Source: CAD feature listing. Evaluate the final solid. Frame: model axes, mm. A direction names the side the tool comes from. Give positions to 0.01 mm unless a question says otherwise; leave off trailing zeros. Write each loop counter-clockwise with the first axis right and the second up, starting at its lowest first coordinate (ties: lowest second). Pieces come first, ordered by that corner, then holes. Notation, with made-up numbers: (-31, -16.75) - (-26, -16.75) arc R20 ccw to (-26, -5.75) - close; hole circle Ø8 at (39, 46.5). An arc over 180 degrees is marked (long way). One line per question, with ' | ' between items. Start each with the question number.
(1) Draft query along Z for faces 5 (the flat face through (-57, -19, 0)), 6 (the flat face through (-39, -57, 5)), 7 (the cylindrical face through (-2.9, -4.34, -17.46)). Return one class per face: +Z half, -Z half, draft (parallel to the pull), parting line (faces both ways), or undercut.
(2) Access query for faces 1 (the flat face through (-30, -30, -15)), 2 (the flat face through (-30, -60, 2)), 3 (the cylindrical face through (-6.99, -47.65, -7.4)), 4 (the flat face through (-30, -30, 0)). Directions: +Z, -Z, +X, -X, +Y, -Y. A direction counts if a zero-diameter tool reaches every point of the face in a straight line with its end or side. Return the directions, or none.
(3) Section A-A, the plane y = -30. Return loops of the section in (x, z), plus the area to 3 significant figures.
(4) Pin query (flat end, axial travel): pin 1 (3 mm diameter, centred on x = -47, y = -31, fed in from -Z); pin 2 (2.5 mm diameter, centred on x = -55, y = -55, fed in from +Z); pin 3 (3 mm diameter, centred on x = -9.5, z = -11, fed in from +Y); pin 4 (1.5 mm diameter, centred on x = -38.5, z = -12, fed in from +Y). Return the tip coordinate at first contact, or that it passes through.
(5) Section D-D, the plane z = -3. Return loops of the section in (x, y).
(6) Section B-B, the plane z = 2. Return loops of the section in (x, y), plus the area to 3 significant figures.
(7) Ray query, line 1 (Y direction, x = -4.5, z = 3.75); line 2 (Y direction, x = -30, z = -17.6); line 3 (Y direction, x = -55, z = -17.1). Return the intervals inside material, ascending. Write a range as [from, to].
```python
from build123d import *

# Parameters (mm, degrees)
SKETCH_1_W          = 60
SKETCH_1_H          = 60
EXTRUDE_1_DEPTH     = 5
SKETCH_3_R          = 29
EXTRUDE_2_DEPTH     = 15
SKETCH_4_W          = 60
SKETCH_4_H          = 60
EXTRUDE_3_DEPTH     = 5
FILLET_1_R          = 5
SKETCH_5_R          = 2.2
CUT_EXTRUDE_1_DEPTH = 89.459030065
SKETCH_6_R          = 28
CUT_EXTRUDE_4_DEPTH = 5
CUT_EXTRUDE_START   = -5
SKETCH_7_R          = 28
CUT_EXTRUDE_5_DEPTH = 5


with BuildPart() as part:
    # Sketch 1 → Extrude 1 (new body)
    with BuildSketch(Plane.XY):
        with Locations((-30, -30)):
            Rectangle(SKETCH_1_W, SKETCH_1_H)
    extrude(amount=EXTRUDE_1_DEPTH)

    # Sketch 3 → Extrude 2 (add)
    with BuildSketch(Plane(origin=(0, 0, 0), x_dir=(-1, 0, 0), z_dir=(0, 0, -1))):
        with Locations((30, -30)):
            Circle(SKETCH_3_R)
    extrude(amount=EXTRUDE_2_DEPTH)

    # Sketch 4 → Extrude 3 (add)
    with BuildSketch(Plane(origin=(0, 0, -15), x_dir=(-1, 0, 0), z_dir=(0, 0, -1))):
        with Locations((30, -30)):
            Rectangle(SKETCH_4_W, SKETCH_4_H)
    extrude(amount=EXTRUDE_3_DEPTH)

    # Fillet 1
    fillet_1_edges = [part.edges().sort_by_distance(p)[0] for p in [
        (0, 0, -17.5),
        (0, -60, -17.5),
        (-60, -60, -17.5),
        (-60, 0, -17.5),
        (0, -60, 2.5),
        (-60, -60, 2.5),
        (-60, 0, 2.5),
        (0, 0, 2.5),
    ]]
    fillet(fillet_1_edges, radius=FILLET_1_R)

    # Sketch 5 → Cut-Extrude 1 (cut, through all)
    with BuildSketch(Plane.XY.offset(5)):
        with Locations((-55, -5)):
            Circle(SKETCH_5_R)
        with Locations((-5, -5)):
            Circle(SKETCH_5_R)
        with Locations((-5, -55)):
            Circle(SKETCH_5_R)
        with Locations((-55, -55)):
            Circle(SKETCH_5_R)
    extrude(amount=-CUT_EXTRUDE_1_DEPTH, mode=Mode.SUBTRACT)

    # Sketch 6 → Cut-Extrude 4 (cut)
    with BuildSketch(Plane(origin=(0, 0, -20), x_dir=(-1, 0, 0), z_dir=(0, 0, -1))):
        with Locations((30, -30)):
            Circle(SKETCH_6_R)
    extrude(amount=-CUT_EXTRUDE_4_DEPTH, mode=Mode.SUBTRACT)

    # Sketch 7 → Cut-Extrude 5 (cut)
    with BuildSketch(Plane.XY.offset(5).offset(CUT_EXTRUDE_START)):
        with Locations(Location((-30, -30, 0), (0, 0, 180))):
            Circle(SKETCH_7_R)
    extrude(amount=CUT_EXTRUDE_5_DEPTH, mode=Mode.SUBTRACT)


solid = part.part
```
Check sheet entries:
1) face 5: undercut | face 6: +Z half | face 7: draft
2) face 1: -Z | face 2: +Z, -Z, +X, -X, -Y | face 3: none | face 4: +Z
3) outline: (-60, -20) - (-58, -20) - (-58, -15) - (-2, -15) - (-2, -20) - (0, -20) - (0, -15) - (-1, -15) - (-1, 0) - (0, 0) - (0, 5) - (-2, 5) - (-2, 0) - (-58, 0) - (-58, 5) - (-60, 5) - (-60, 0) - (-59, 0) - (-59, -15) - (-60, -15) - close | area: 910 mm²
4) pin 1: z = -15 | pin 2: through | pin 3: y = -8.09 | pin 4: y = -2.05
5) outline: circle Ø58 at (-30, -30)
6) outline: (-60, -55) arc R5 ccw to (-55, -60) - (-5, -60) arc R5 ccw to (0, -55) - (0, -5) arc R5 ccw to (-5, 0) - (-55, 0) arc R5 ccw to (-60, -5) - close; hole circle Ø56 at (-30, -30); hole circle Ø4.4 at (-55, -55); hole circle Ø4.4 at (-55, -5); hole circle Ø4.4 at (-5, -55); hole circle Ø4.4 at (-5, -5) | area: 1,050 mm²
7) line 1: [-59.97, -57.14], [-52.86, -41.57], [-18.43, -7.14], [-2.86, -0.03] | line 2: [-60, -58], [-2, 0] | line 3: [-60, -57.2], [-52.8, -42.61], [-17.39, -7.2], [-2.8, 0]
